Here's how the part is built. I have some questions about the finished solid (model axes, mm). A direction names the side the tool comes from. Round coordinates to 2 decimals unless told otherwise and drop trailing zeros. Order: outer loops, then holes, each group sorted by start corner. A loop starts at its lowest first (then second) coordinate and runs counter-clockwise, first axis right, second up. Notation, with made-up numbers: (-17.75, -17) - (17.25, -17) arc R15 ccw to (17.25, -11) - close; hole circle Ø10 at (19.5, 9.25). An arc over 180 degrees is marked (long way). One line per item, written item: value.
from build123d import *

# Parameters (mm, degrees)
SKETCH1_R           = 18.25
BOSS_EXTRUDE1_DEPTH = 12.5
BOSS_EXTRUDE2_START = -2
SKETCH2_R           = 1.75
BOSS_EXTRUDE2_DEPTH = 2
SKETCH3_R           = 8
BOSS_EXTRUDE3_DEPTH = 2
SKETCH4_R           = 2.5
BOSS_EXTRUDE4_DEPTH = 5.5


with BuildPart() as part:
    # Sketch1 → Boss-Extrude1 (new body)
    with BuildSketch(Plane.XY):
        Circle(SKETCH1_R)
    extrude(amount=BOSS_EXTRUDE1_DEPTH)

    # Sketch2 → Boss-Extrude2 (add)
    # profile 1 of 2: a face of its own
    with BuildSketch(Plane.XY.offset(12.5).offset(BOSS_EXTRUDE2_START)):
        with BuildLine():
            Line((-23.407860756, 2.960513809), (-17.235501153, 6))
            ThreePointArc((-17.235501153, 6), (-18.25, 0), (-17.235501153, -6))
            Line((-17.235501153, -6), (-23.407860756, -2.960513809))
            ThreePointArc((-23.407860756, -2.960513809), (-25.25, 0), (-23.407860756, 2.960513809))
        make_face()
        with Locations((-21.95, 0)):
            Circle(SKETCH2_R, mode=Mode.SUBTRACT)
    # profile 2 of 2: a face of its own
    with BuildSketch(Plane.XY.offset(12.5).offset(BOSS_EXTRUDE2_START)):
        with BuildLine():
            Line((23.407860756, 2.960513809), (17.235501153, 6))
            ThreePointArc((17.235501153, 6), (18.25, 0), (17.235501153, -6))
            Line((17.235501153, -6), (23.407860756, -2.960513809))
            ThreePointArc((23.407860756, -2.960513809), (25.25, 0), (23.407860756, 2.960513809))
        make_face()
        with Locations((21.95, 0)):
            Circle(SKETCH2_R, mode=Mode.SUBTRACT)
    extrude(amount=BOSS_EXTRUDE2_DEPTH)

    # Sketch3 → Boss-Extrude3 (add)
    with BuildSketch(Plane.XY.offset(12.5)):
        Circle(SKETCH3_R)
    extrude(amount=BOSS_EXTRUDE3_DEPTH)

    # Sketch4 → Boss-Extrude4 (add)
    with BuildSketch(Plane.XY.offset(14.5)):
        Circle(SKETCH4_R)
    extrude(amount=BOSS_EXTRUDE4_DEPTH)


solid = part.part
Q1. If we section it at D-D, the plane x = 0: Please give me the cut outline in (y, z).
Results list:
outline: (-18.25, 0) - (18.25, 0) - (18.25, 12.5) - (8, 12.5) - (8, 14.5) - (2.5, 14.5) - (2.5, 20) - (-2.5, 20) - (-2.5, 14.5) - (-8, 14.5) - (-8, 12.5) - (-18.25, 12.5) - close
Q2. Will these pins go through, and if not, where does the flat tip stop? pin 1 (6.5 mm diameter, centred on x = 21, y = -1.5, fed in from -Z); pin 2 (5 mm diameter, centred on x = -8, z = 11, fed in from -Y); pin 3 (8 mm diameter, centred on x = 9.5, y = -5.5, fed in from +Z); pin 4 (2.5 mm diameter, centred on x = -23, y = 1.5, fed in from -Z).
Results list:
pin 1: z = 0
pin 2: y = -17.4
pin 3: z = 14.5
pin 4: z = 10.5
Q3. Which directions (+Z, -Z, +X, -X, +Y, -Y) give clear straight access to the entire face, cutting with the end or side of a thin tool? Please do faces 1 (the flat face through (-20.28, -4.5, 11.49)), 2 (the cylindrical face through (8.4, -16.2, 6.2)), 3 (the flat face through (-0.4, 8.4, 12.5)).
Results list:
face 1: +Z, -Z, -X, -Y
face 2: -Z
face 3: +Z
Q4. If we section it at A-A, the plane y = 0: Please give me the cut outline in (x, z), then the cut area to 3 significant figures.
Results list:
outline: (-25.25, 10.5) - (-23.7, 10.5) - (-23.7, 12.5) - (-25.25, 12.5) - close; (-20.2, 10.5) - (-18.25, 10.5) - (-18.25, 0) - (18.25, 0) - (18.25, 10.5) - (20.2, 10.5) - (20.2, 12.5) - (8, 12.5) - (8, 14.5) - (2.5, 14.5) - (2.5, 20) - (-2.5, 20) - (-2.5, 14.5) - (-8, 14.5) - (-8, 12.5) - (-20.2, 12.5) - close; (23.7, 10.5) - (25.25, 10.5) - (25.25, 12.5) - (23.7, 12.5) - close
area: 530 mm²
Q5. If I drill on line 1 along Z through (x, y) = (12.5, 0); line 2 along Y through (x, z) = (-21.95, 11.4); line 3 along Z through (x, y) = (20, -2), over which ranges is the centre line in solid material (lowest first)?
Results list:
line 1: 0 to 12.5
line 2: -3.68 to -1.75, 1.75 to 3.68
line 3: 10.5 to 12.5
Q6. We'd pull the mould along Y, two halves only. Please class faces 4 (the cylindrical face through (-20.281, 0.526, 11.486)), 5 (the cylindrical face through (25.25, -0.05, 11.49)), 6 (the flat face through (-20, -1, 10.5)): released by +Y, released by -Y, zero draft, split by the parting line, or undercut.
Results list:
face 4: undercut
face 5: split by the parting line
face 6: zero draft
Q7. If we section it at B-B, the plane z = 11.5: Please give me the cut outline in (x, y).
Results list:
outline: (-23.41, -2.96) - (-17.24, -6) arc R18.25 ccw to (17.24, -6) - (23.41, -2.96) arc R3.3 ccw to (23.41, 2.96) - (17.24, 6) arc R18.25 ccw to (-17.24, 6) - (-23.41, 2.96) arc R3.3 ccw to start; hole circle Ø3.5 at (-21.95, 0); hole circle Ø3.5 at (21.95, 0)
Q8. If we section it at C-C, the plane x = 21.95: Please give me the cut outline in (y, z), then the cut area to 3 significant figures.
Results list:
outline: (-3.68, 10.5) - (-1.75, 10.5) - (-1.75, 12.5) - (-3.68, 12.5) - close; (1.75, 10.5) - (3.68, 10.5) - (3.68, 12.5) - (1.75, 12.5) - close
area: 7.71 mm²
